```python
from build123d import *

# Parameters (mm, degrees)
SKETCH2_W           = 50
SKETCH2_H           = 16
BOSS_EXTRUDE1_DEPTH = 17.5
SKETCH3_R           = 8
CUT_EXTRUDE1_DEPTH  = 182.811028268
BOSS_EXTRUDE2_START = -3
SKETCH4_W           = 16
SKETCH4_H           = 3
BOSS_EXTRUDE2_DEPTH = 43
FILLET1_R           = 0.5
FILLET2_R           = 6
SKETCH6_R           = 3
CUT_EXTRUDE3_DEPTH  = 12
BOSS_EXTRUDE3_DEPTH = 4
BOSS_EXTRUDE5_START = -35
BOSS_EXTRUDE5_DEPTH = 4
SKETCH8_W           = 27
SKETCH8_H           = 52
SKETCH8_R           = 10
BOSS_EXTRUDE6_DEPTH = 4
CHAMFER1_SIZE2      = 4
CHAMFER1_SIZE       = 3
SKETCH9_W           = 27
SKETCH9_H           = 98.792712282
BOSS_EXTRUDE7_DEPTH = 4
CHAMFER2_SIZE       = 2


with BuildPart() as part:
    # Sketch1 → Revolve1 (revolve)
    with BuildSketch(Plane(origin=(0, 0, 0), x_dir=(0, 0, -1), z_dir=(1, 0, 0))):
        Polygon((8, 157), (8, 0), (10, 0), (10, 4), (12, 4), (12, 7), (10, 7), (10, 157), align=None)
    revolve(axis=Axis((0, 0, 0), (0, 1, 0)))



with BuildPart() as body_2:
    # Sketch2 → Boss-Extrude1 (new, symmetric)
    with BuildSketch(Plane(origin=(0, 0, 0), x_dir=(0, 0, -1), z_dir=(1, 0, 0))):
        with Locations((53, -96)):
            Rectangle(SKETCH2_W, SKETCH2_H)
    extrude(amount=BOSS_EXTRUDE1_DEPTH, both=True)

    # Sketch3 → Cut-Extrude1 (cut, through all)
    with BuildSketch(Plane(origin=(0, 0, -78), x_dir=(-1, 0, 0), z_dir=(0, 0, -1))):
        with Locations((0, -104)):
            Circle(SKETCH3_R)
    extrude(amount=-CUT_EXTRUDE1_DEPTH, mode=Mode.SUBTRACT)

    # Sketch4 → Boss-Extrude2 (add)
    with BuildSketch(Plane(origin=(0, 0, -78), x_dir=(-1, 0, 0), z_dir=(0, 0, -1)).offset(BOSS_EXTRUDE2_START)):
        with Locations((0, -97.5)):
            Rectangle(SKETCH4_W, SKETCH4_H)
    extrude(amount=-BOSS_EXTRUDE2_DEPTH)

    # Fillet1
    fillet1_edges = [body_2.edges().sort_by_distance(p)[0] for p in [
        (0, -99, -32),
        (0, -99, -75),
    ]]
    fillet(fillet1_edges, radius=FILLET1_R)

    # Fillet2
    fillet2_edges = [body_2.edges().sort_by_distance(p)[0] for p in [
        (0, -88, -78),
    ]]
    fillet(fillet2_edges, radius=FILLET2_R)

    # Sketch6 → Cut-Extrude3 (cut)
    with BuildSketch(Plane.XZ.offset(104)):
        with Locations(Location((-12.5, -34, 0), (0, 0, 270))):
            Circle(SKETCH6_R)
        with Locations(Location((12.5, -34, 0), (0, 0, 270))):
            Circle(SKETCH6_R)
        with Locations(Location((-12.5, -72, 0), (0, 0, 270))):
            Circle(SKETCH6_R)
        with Locations(Location((12.5, -72, 0), (0, 0, 270))):
            Circle(SKETCH6_R)
    extrude(amount=-CUT_EXTRUDE3_DEPTH, mode=Mode.SUBTRACT)


with BuildPart() as body_3:
    # Sketch7 → Boss-Extrude3 (new body)
    with BuildSketch(Plane.ZY.offset(17.5)):
        with BuildLine():
            Line((-72, -88), (-36, 4))
            Line((-36, 4), (16, 4))
            Line((16, 4), (16, -5))
            Line((16, -5), (-2, -5))
            ThreePointArc((-2, -5), (-20.384776311, -12.615223689), (-28, -31))
            Line((-28, -31), (-28, -88))
            Line((-28, -88), (-72, -88))
        make_face()
    extrude(amount=-BOSS_EXTRUDE3_DEPTH)


with BuildPart() as body_4:
    # Sketch7<2> → Boss-Extrude5 (new body)
    with BuildSketch(Plane.ZY.offset(17.5).offset(BOSS_EXTRUDE5_START)):
        with BuildLine():
            Line((-72, -88), (-36, 4))
            Line((-36, 4), (16, 4))
            Line((16, 4), (16, -5))
            Line((16, -5), (-2, -5))
            ThreePointArc((-2, -5), (-20.384776311, -12.615223689), (-28, -31))
            Line((-28, -31), (-28, -88))
            Line((-28, -88), (-72, -88))
        make_face()
    extrude(amount=BOSS_EXTRUDE5_DEPTH)


with BuildPart() as part_1:
    add(part.part)

    add(body_3.part)  # Boss-Extrude6 merges body 3

    add(body_4.part)  # Boss-Extrude6 merges body 4
    # Sketch8 → Boss-Extrude6 (add)
    with BuildSketch(Plane.XZ.offset(-4)):
        with Locations((0, -10)):
            Rectangle(SKETCH8_W, SKETCH8_H)
        with Locations(Location((0, 0, 0), (0, 0, 270))):
            Circle(SKETCH8_R, mode=Mode.SUBTRACT)
    extrude(amount=BOSS_EXTRUDE6_DEPTH)

    # Chamfer1
    chamfer1_edges = [part_1.edges().sort_by_distance(p)[0] for p in [
        (0, 0, -36),
    ]]
    chamfer1_side = [part_1.faces().sort_by_distance(p)[0] for p in [
        (0, 0, -35.94),
    ]]
    chamfer(chamfer1_edges, length=CHAMFER1_SIZE - 0.0001, length2=CHAMFER1_SIZE2 - 0.0001, reference=chamfer1_side[0])  # a hair under: the kernel refuses the full size


    add(body_2.part)  # Boss-Extrude7 merges body 2
    # Sketch9 → Boss-Extrude7 (add)
    with BuildSketch(Plane(origin=(0, 12.747540984, -32.57704918), x_dir=(-1, 0, 0), z_dir=(0, 0.3643993485805124, -0.9312427797057534))):
        with Locations((0, -58.789761571)):
            Rectangle(SKETCH9_W, SKETCH9_H)
    extrude(amount=-BOSS_EXTRUDE7_DEPTH)

    # Chamfer2
    chamfer2_edges = [part_1.edges().sort_by_distance(p)[0] for p in [
        (0, 4, 12),
    ]]
    chamfer(chamfer2_edges, length=CHAMFER2_SIZE)


solid = part_1.part
```
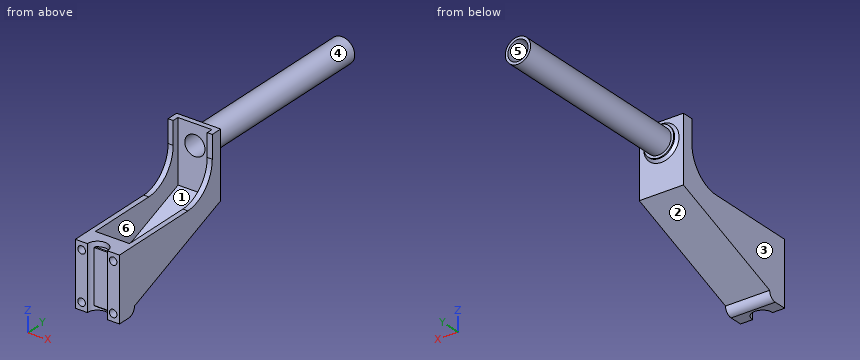
Verification items for the finished model (mm, model axes). Face numbers are marked on the shaded views. A direction names the side the tool comes from. Round coordinates to 2 decimals unless told otherwise and drop trailing zeros. Order: outer loops, then holes, each group sorted by start corner. A loop starts at its lowest first (then second) coordinate and runs counter-clockwise, first axis right, second up. Notation, with made-up numbers: (58.5, -26.5) - (112.5, -26.5) arc R25 cw to (112.5, -12.5) - close; hole circle Ø11 at (30.5, 56.5). An arc over 180 degrees is marked (long way). Use CSV: the item, a comma, the result in double quotes. Start each with the question number.
1) Section check D-D, the plane z = -20. Record the cut outline in (x, y).
2) Go/stop test with flat-tipped pins: P1, Ø3, axis at x = 16, z = 11, coming from the -Y side; P2, Ø1.8, axis at x = 13, z = -34, coming from the -Y side; P3, Ø8, axis at x = 3, z = -6.5, coming from the -Y side; P4, Ø9.5, axis at x = 0, z = 0, coming from the -Y side. Record where each tip stops, or that it passes through.
3) Mould release check, pull along X, two halves, no side actions. Record for the marked faces 1, 2 and 3: +X half, -X half, draft (parallel to the pull), parting line (faces both ways), or undercut.
4) Section check B-B, the plane y = 40. Record the cut outline in (x, z), plus the area to 3 significant figures.
5) Section check C-C, the plane z = -63. Record the cut outline in (x, y) (3 decimals).
6) Access from +Z, -Z, +X, -X, +Y, -Y to the whole of each face (thin tool, end or side, straight path). Record for the marked faces 4, 5 and 6.
7) Thickness scan on L1, parallel to Z at x = 12, y = -96; L2, parallel to X at y = -97.5, z = -34; L3, parallel to Y at x = 0.5, z = -32.5. Record the ranges inside material, lowest first.
Answers:
1,outline,"(-17.5, -12.24) - (-13.5, -12.24) - (-13.5, 0) - (13.5, 0) - (13.5, -12.24) - (17.5, -12.24) - (17.5, 4) - (-17.5, 4) - close"
2,P1,"stops at y = -5"
2,P2,"stops at y = -92"
2,P3,"stops at y = 0"
2,P4,"passes through"
3,face 1,"undercut"
3,face 2,"draft"
3,face 3,"-X half"
4,outline,"circle Ø20 at (0, 0); hole circle Ø16 at (0, 0)"
4,area,"113 mm²"
5,outline,"(-17.5, -104) - (-8, -104) arc R8 cw to (-6.245, -99) - (6.245, -99) arc R8 cw to (8, -104) - (17.5, -104) - (17.5, -65) - (-17.5, -65) - close; hole (-13.5, -88) - (13.5, -88) - (13.5, -75.977) - (-13.5, -75.977) - close"
6,face 4,"+Y"
6,face 5,"+Y, -Y"
6,face 6,"+Z"
7,L1,"z = -78 to -74.96, -69.04 to -36.96, -31.04 to -28"
7,L2,"x = -17.5 to -15.5, -9.5 to 9.5, 15.5 to 17.5"
7,L3,"y = -99 to -88, 0 to 4"
